Design review of the part built by this model. Coordinates are the model's own, in mm. Face numbers are marked on the shaded views. A direction names the side the tool comes from. Coordinates: 2 decimals unless noted, no trailing zeros. Write each loop counter-clockwise with the first axis right and the second up, starting at its lowest first coordinate (ties: lowest second). Pieces come first, ordered by that corner, then holes. Notation, with made-up numbers: M -40,87 L 15,87 A35 ccw 15,125 Z; hole C 17.25,43.5 d1. An arc over 180 degrees is marked long. Write item = value, one per line.
```python
from build123d import *

# Parameters (mm, degrees)
SKETCH1_W               = 2.032
SKETCH1_H               = 25.146
CUT_EXTRUDE1_REACH      = 26.41
CUT_EXTRUDE1_END_RADIUS = 1.524
SKETCH2_R               = 0.5715
CIRPATTERN1_COUNT       = 8
SKETCH3_R               = 3.556
SKETCH3_R_2             = 1.524
BOSS_EXTRUDE1_DEPTH     = 6.35
BOSS_EXTRUDE2_START     = 6.35
SKETCH4_R               = 17.78
SKETCH4_R_2             = 1.524
BOSS_EXTRUDE2_DEPTH     = 6.35
CUT_EXTRUDE2_REACH      = 47.438
SKETCH11_R              = 1.63195
CIRPATTERN2_COUNT       = 6
CHAMFER1_SIZE           = 3.048
CHAMFER1_SIZE2          = 5.279290861
SKETCH13_R              = 11.43
SKETCH13_R_2            = 6.54812
BOSS_EXTRUDE4_DEPTH     = 12.7
FILLET4_R               = 0.254
CHAMFER2_SIZE           = 0.851662
CHAMFER2_SIZE2          = 0.83947
BOSS_EXTRUDE5_START     = 6.35
SKETCH15_R              = 4.699
SKETCH15_R_2            = 3.556
BOSS_EXTRUDE5_DEPTH     = 6.35


with BuildPart() as part:
    # Sketch1 → Revolve2 (revolve)
    with BuildSketch(Plane.XY, mode=Mode.PRIVATE) as revolve2_sk:
        with Locations((-2.54, 10.505774136)):
            Rectangle(SKETCH1_W, SKETCH1_H)
    revolve(revolve2_sk.sketch.rotate(Axis((0, 8.215698649, 0), (0, -1, 0)), 270), axis=Axis((0, 8.215698649, 0), (0, -1, 0)))

    # Cut-Extrude1: up to this cylinder (the profile starts outside it)
    cut_extrude1_end = Plane(origin=(0, -0.543226, 0), z_dir=(0, 1, 0)) * Cylinder(CUT_EXTRUDE1_END_RADIUS, 56.868, mode=Mode.PRIVATE)
    # Sketch2 → Cut-Extrude1 (cut, up to the surface)
    with BuildSketch(Plane.ZY.offset(3.556), mode=Mode.PRIVATE) as cut_extrude1_sk1:
        with Locations((0.000240101, -0.543225864)):
            Circle(SKETCH2_R)
    cut_extrude1_tool1 = extrude(cut_extrude1_sk1.sketch, amount=-CUT_EXTRUDE1_REACH, mode=Mode.PRIVATE) - cut_extrude1_end
    cut_extrude1 = cut_extrude1_tool1.solids().sort_by_distance((-3.556, -0.543226, 0.00024))[0]
    add(cut_extrude1, mode=Mode.SUBTRACT)

    # CirPattern1: Cut-Extrude1 ×8 about axis
    cirpattern1_axis = Axis((0, -2.067225864, 0), (0, 1, 0))
    for i in range(1, CIRPATTERN1_COUNT):
        add(cut_extrude1.rotate(cirpattern1_axis, i * 360 / CIRPATTERN1_COUNT), mode=Mode.SUBTRACT)

    # Sketch3 → Boss-Extrude1 (add)
    with BuildSketch(Plane(origin=(0, 23.078774136, 0), x_dir=(-1, 0, 0), z_dir=(0, -1, 0))):
        with Locations(Location((0, 0, 0), (0, 0, 270))):
            Circle(SKETCH3_R)
        with Locations(Location((0, 0, 0), (0, 0, 270))):
            Circle(SKETCH3_R_2, mode=Mode.SUBTRACT)
    extrude(amount=-BOSS_EXTRUDE1_DEPTH)

    # Sketch4 → Boss-Extrude2 (add)
    with BuildSketch(Plane(origin=(0, 29.428774136, 0), x_dir=(1, 0, 0), z_dir=(0, 1, 0)).offset(BOSS_EXTRUDE2_START)):
        with Locations(Location((0, 0, 0), (0, 0, 270))):
            Circle(SKETCH4_R)
        with Locations(Location((0, 0, 0), (0, 0, 270))):
            Circle(SKETCH4_R_2, mode=Mode.SUBTRACT)
    extrude(amount=-BOSS_EXTRUDE2_DEPTH)

    # Sketch11 → Cut-Extrude2 (cut, up to next)
    with BuildSketch(Plane(origin=(0, 35.778774136, 0), x_dir=(1, 0, 0), z_dir=(0, 1, 0)), mode=Mode.PRIVATE) as cut_extrude2_sk1:
        with Locations(Location((0, -15.24, 0), (0, 0, 270))):
            Circle(SKETCH11_R)
    cut_extrude2_tool1 = extrude(cut_extrude2_sk1.sketch, amount=-CUT_EXTRUDE2_REACH, mode=Mode.PRIVATE) & part.part
    cut_extrude2 = cut_extrude2_tool1.solids().sort_by_distance((0, 35.778774, 15.24))[0]
    add(cut_extrude2, mode=Mode.SUBTRACT)

    # CirPattern2: Cut-Extrude2 ×6 about axis
    cirpattern2_axis = Axis((0, 0, 0), (0, 1, 0))
    for i in range(1, CIRPATTERN2_COUNT):
        add(cut_extrude2.rotate(cirpattern2_axis, i * 360 / CIRPATTERN2_COUNT), mode=Mode.SUBTRACT)

    # Chamfer1
    chamfer1_edges = [part.edges().sort_by_distance(p)[0] for p in [
        (0, 35.778774136, -1.524),
    ]]
    chamfer1_side = [part.faces().sort_by_distance(p)[0] for p in [
        (0, 35.778774136, -17.277105657),
    ]]
    chamfer(chamfer1_edges, length=CHAMFER1_SIZE, length2=CHAMFER1_SIZE2, reference=chamfer1_side[0])

    # Sketch13 → Boss-Extrude4 (add)
    with BuildSketch(Plane(origin=(0, 35.778774136, 0), x_dir=(1, 0, 0), z_dir=(0, 1, 0))):
        with Locations(Location((0, 0, 0), (0, 0, 270))):
            Circle(SKETCH13_R)
        with Locations(Location((0, 0, 0), (0, 0, 270))):
            Circle(SKETCH13_R_2, mode=Mode.SUBTRACT)
    extrude(amount=BOSS_EXTRUDE4_DEPTH)

    # Fillet4
    fillet4_edges = [part.edges().sort_by_distance(p)[0] for p in [
        (0, 35.778774136, -11.43),
    ]]
    fillet(fillet4_edges, radius=FILLET4_R)

    # Chamfer2
    chamfer2_edges = [part.edges().sort_by_distance(p)[0] for p in [
        (0, 48.478774136, -6.54812),
    ]]
    chamfer2_side = [part.faces().sort_by_distance(p)[0] for p in [
        (0, 48.478774136, -11.10671078),
    ]]
    chamfer(chamfer2_edges, length=CHAMFER2_SIZE, length2=CHAMFER2_SIZE2, reference=chamfer2_side[0])

    # Sketch15 → Boss-Extrude5 (add)
    with BuildSketch(Plane.XZ.offset(-29.428774136).offset(BOSS_EXTRUDE5_START)):
        with Locations(Location((0, 0, 0), (0, 0, 90))):
            Circle(SKETCH15_R)
        with Locations(Location((0, 0, 0), (0, 0, 90))):
            Circle(SKETCH15_R_2, mode=Mode.SUBTRACT)
    extrude(amount=-BOSS_EXTRUDE5_DEPTH)


solid = part.part
```
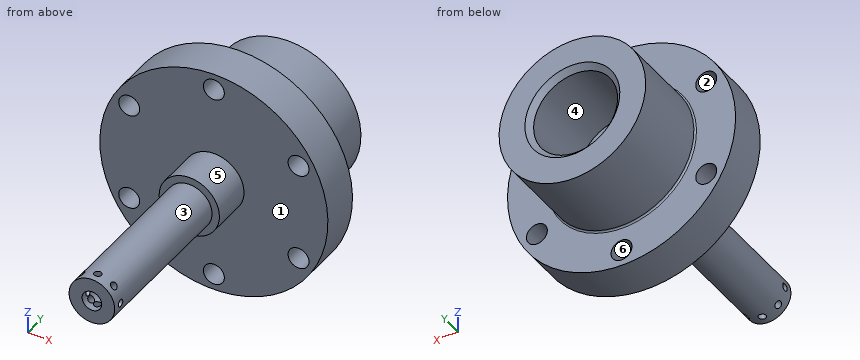
Q1. Consider section B-B, the plane y = 34. State the section outline as (x, z) points.
Check result:
outline = C 0,0 d35.56; hole C -13.2,-7.62 d3.26; hole C -13.2,7.62 d3.26; hole C 0,0 d7.09; hole C 0,-15.24 d3.26; hole C 0,15.24 d3.26; hole C 13.2,-7.62 d3.26; hole C 13.2,7.62 d3.26
Q2. The part is to be moulded in two halves that separate along X. For the marked faces 1, 2 and 3, say which applies: +X half, -X half, draft (parallel to the pull), parting line (faces both ways), or undercut.
Check result:
face_1 = draft
face_2 = undercut
face_3 = parting line
Q3. Consider section C-C, the plane x = -14. State the section outline as (y, z) points.
Check result:
outline = M 29.43,-10.96 L 35.78,-10.96 L 35.78,-9.04 L 29.43,-9.04 Z; M 29.43,-6.2 L 35.78,-6.2 L 35.78,6.2 L 29.43,6.2 Z; M 29.43,9.04 L 35.78,9.04 L 35.78,10.96 L 29.43,10.96 Z
Q4. Wall thickness on line 1 (X direction, y = 33.5, z = 7.62); line 2 (X direction, y = 9, z = 0); line 3 (X direction, y = 32, z = 8): over which ranges is each line inside the solid? List them lowest first.
Check result:
line_1 = -16.06 to -14.83, -11.57 to 11.57, 14.83 to 16.06
line_2 = -3.56 to -1.52, 1.52 to 3.56
line_3 = -15.88 to -14.79, -11.61 to 11.61, 14.79 to 15.88
Q5. Consider section D-D, the plane z = 15.24. State the section outline as (x, y) points.
Check result:
outline = M -9.16,29.43 L -1.63,29.43 L -1.63,35.78 L -9.16,35.78 Z; M 1.63,29.43 L 9.16,29.43 L 9.16,35.78 L 1.63,35.78 Z
Q6. Machinability: for the marked faces 4, 5 and 6, which of the approach directions +Z, -Z, +X, -X, +Y, -Y give a long, thin tool a straight path to every point of the face, cutting with its end or side? Answer none if there is none.
Check result:
face_4 = +Y
face_5 = -Y
face_6 = +Y, -Y
Q7. Consider section A-A, the plane z = -15. State the section outline as (x, y) points, and give its area (3 significant figures).
Check result:
outline = M -9.55,29.43 L -1.61,29.43 L -1.61,35.78 L -9.55,35.78 Z; M 1.61,29.43 L 9.55,29.43 L 9.55,35.78 L 1.61,35.78 Z
area = 101 mm²
Q8. For P1, Ø1.3, axis at y = -0.54, z = 0, coming from the +X side; P2, Ø8, axis at x = 7, y = 24.5, coming from the -Z side; P3, Ø10.5, axis at x = 1, z = 0, coming from the +Y side, all flat-tipped, find the tip position at first contact; note any pin that passes through.
Check result:
P1 = 3.56
P2 = -3.62
P3 = 35.78
